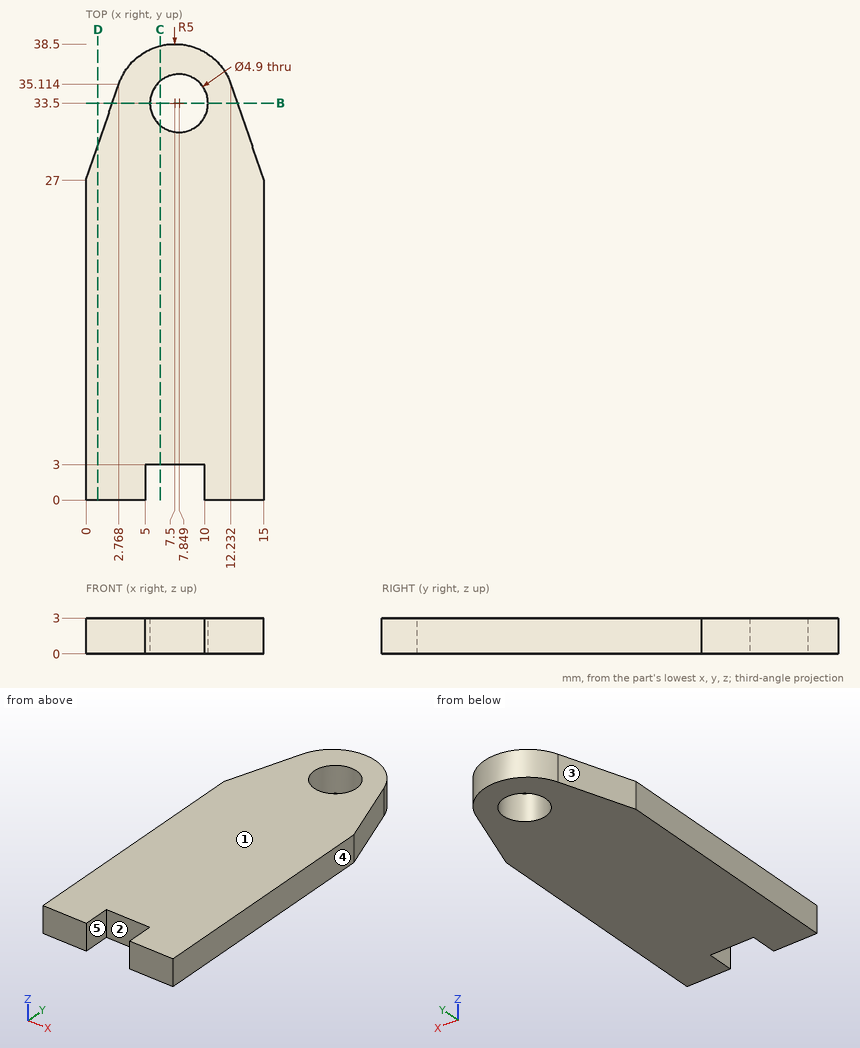
The drawing under review shows one solid part. Ordinate dimensions are in mm from its lowest x, y, z. A direction names the side the tool comes from. Coordinates: 2 decimals unless noted, no trailing zeros. Order: outer loops, then holes, each group sorted by start corner. A loop starts at its lowest first (then second) coordinate and runs counter-clockwise, first axis right, second up. Notation, with made-up numbers: (48, -34.75) - (52, -34.75) arc R20 cw to (52, -11.75) - close; hole circle Ø10 at (67.25, 38). An arc over 180 degrees is marked (long way). Put each result on its own line as item: value.
1) Tool access review of the marked faces 4 and 5: name each direction out of +Z, -Z, +X, -X, +Y, -Y from which nothing blocks a thin tool from reaching the whole face with its end or side.
Response values:
face 4: +Z, -Z, +X, +Y, -Y
face 5: +Z, -Z, -Y
2) Take a section at D-D, the plane x = 1. Give the boundary of the cut face in (y, z).
Response values:
outline: (0, 0) - (29.93, 0) - (29.93, 3) - (0, 3) - close
3) Insertion check: P1, Ø1.5, axis at y = 2, z = 2, coming from the -X side. The pin has a flat end and moves straight along its axis. Give the tip position at first contact, or say it passes through.
Response values:
P1: stops at x = 0
4) The part is to be moulded in two halves that separate along X. For the marked faces 1, 2 and 3, say which applies: released by +X, released by -X, zero draft, split by the parting line, or undercut.
Response values:
face 1: zero draft
face 2: undercut
face 3: released by -X
5) Take a section at C-C, the plane x = 6.25. Give the boundary of the cut face in (y, z).
Response values:
outline: (3, 0) - (31.64, 0) - (31.64, 3) - (3, 3) - close; (35.36, 0) - (38.34, 0) - (38.34, 3) - (35.36, 3) - close
6) Wall thickness on L1, parallel to Y at x = 7.75, z = 2.25; L2, parallel to Y at x = 8.5, z = 1.85; L3, parallel to Y at x = 11.75, z = 1 (1 decimal): over which ranges is each line inside the solid? List them lowest first. Write a range as from..to.
Response values:
L1: y = 3..31.05, 35.95..38.49
L2: y = 3..31.14, 35.86..38.4
L3: y = 0..36.1
7) Take a section at B-B, the plane y = 33.5. Give the boundary of the cut face in (x, z).
Response values:
outline: (2.22, 0) - (5.4, 0) - (5.4, 3) - (2.22, 3) - close; (10.3, 0) - (12.78, 0) - (12.78, 3) - (10.3, 3) - close
